Part print with two shaded views. Sizes in mm from the minimum x, y, z corner. A direction names the side the tool comes from. Coordinates: 2 decimals unless noted, no trailing zeros. Order: outer loops, then holes, each group sorted by start corner. A loop starts at its lowest first (then second) coordinate and runs counter-clockwise, first axis right, second up. Notation, with made-up numbers: (-24.5, 9.25) - (-2.5, 9.25) arc R34 ccw to (-2.5, 43.25) - close; hole circle Ø10 at (19.25, -21). An arc over 180 degrees is marked (long way). One line per item, written item: value.
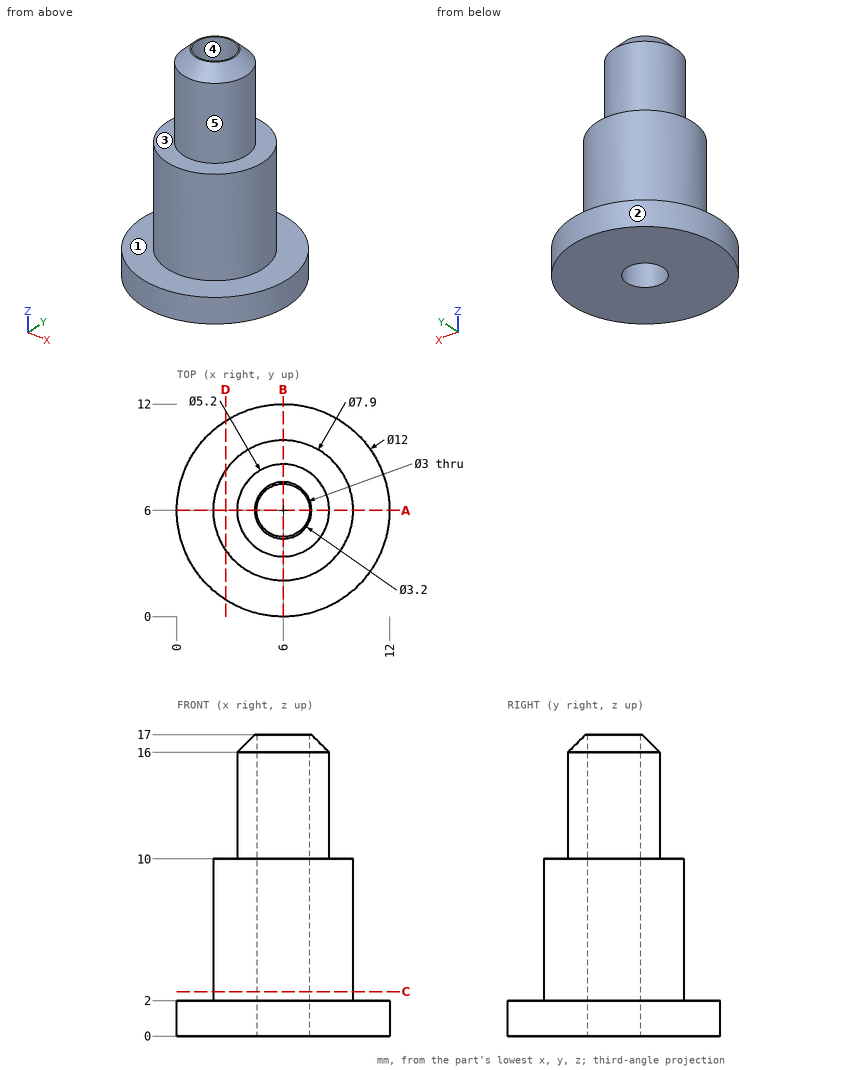
1. 3-axis set-ups, long thin cutter, end or side, ignore diameter. For the marked faces 1 and 2: which of +Z, -Z, +X, -X, +Y, -Y reach the whole face in a straight line?
Values found:
face 1: +Z
face 2: +Z, -Z
2. Band-saw the part on C-C, the plane z = 2.5. Give the cut face in (x, y), and give its area (3 significant figures).
Values found:
outline: circle Ø7.9 at (6, 6); hole circle Ø3 at (6, 6)
area: 41.9 mm2
3. Probe line 1 along Y through (x, z) = (6, 8.25); line 2 along Y through (x, z) = (6, 10.5); line 3 along Z through (x, y) = (2.5, 7). List the from-to ranges inside material, lowest first.
Values found:
line 1: y = 2.05 to 4.5, 7.5 to 9.95
line 2: y = 3.4 to 4.5, 7.5 to 8.6
line 3: z = 0 to 10
4. Band-saw the part on D-D, the plane x = 2.75. Give the cut face in (y, z) (3 decimals), and give its area (3 significant figures).
Values found:
outline: (0.956, 0) - (11.044, 0) - (11.044, 2) - (8.245, 2) - (8.245, 10) - (3.755, 10) - (3.755, 2) - (0.956, 2) - close
area: 56.1 mm2
5. Two-plate mould, pull along Y, no slides. Class the marked faces 3, 4 and 5: pulls with the +Y half, pulls with the -Y half, needs draft (parallel to the pull), parting line crosses it, or undercut.
Values found:
face 3: needs draft
face 4: undercut
face 5: parting line crosses it
6. Band-saw the part on A-A, the plane y = 6. Give the cut face in (x, z).
Values found:
outline: (0, 0) - (4.5, 0) - (4.5, 17) - (4.4, 17) - (3.4, 16) - (3.4, 10) - (2.05, 10) - (2.05, 2) - (0, 2) - close; (7.5, 0) - (12, 0) - (12, 2) - (9.95, 2) - (9.95, 10) - (8.6, 10) - (8.6, 16) - (7.6, 17) - (7.5, 17) - close
7. Flat gauge pins, fed straight in: P1, Ø2, axis at x = 5.5, z = 13, coming from the -Y side; P2, Ø2, axis at y = 4.5, z = 15, coming from the +X side; P3, Ø1, axis at y = 9.5, z = 5.5, coming from the -X side; P4, Ø4, axis at x = 6, y = 6, coming from the -Z side. Where does each tip first touch, or does it go through?
Values found:
P1: stops at y = 3.4
P2: stops at x = 8.55
P3: stops at x = 3.43
P4: stops at z = 0
